from build123d import *

# Parameters (mm, degrees)
BOSS_EXTRUDE1_DEPTH = 60


with BuildPart() as part:
    # Sketch1 → Boss-Extrude1 (new body)
    with BuildSketch(Plane(origin=(0, 0, 0), x_dir=(1, 0, 0), z_dir=(0, 1, 0))):
        with BuildLine():
            Line((-38.729833462, -10), (-20.877867157, -79.140368196))
            Line((-20.877867157, -79.140368196), (-44.722080497, -147.638269612))
            ThreePointArc((-44.722080497, -147.638269612), (-42.5, -153.612159322), (-36.215419503, -152.549592626))
            Line((-36.215419503, -152.549592626), (15.138321986, -93.070241293))
            ThreePointArc((15.138321986, -93.070241293), (17.71723932, -89.278977901), (19.364916731, -85))
            Line((19.364916731, -85), (38.729833462, -10))
            ThreePointArc((38.729833462, -10), (0, 40), (-38.729833462, -10))
        make_face()
    extrude(amount=BOSS_EXTRUDE1_DEPTH)


solid = part.part
Geometry: final body of the model. Coordinates: model frame, mm. A direction names the side the tool comes from. Give positions to 0.01 mm unless a question says otherwise; leave off trailing zeros. Write each loop counter-clockwise with the first axis right and the second up, starting at its lowest first coordinate (ties: lowest second). Pieces come first, ordered by that corner, then holes. Notation, with made-up numbers: M -24,55 L 15,55 A19 ccw 15,82 Z; hole C 9.25,-39.5 d5. An arc over 180 degrees is marked long. Answer in a Markdown table with one row per item. Add a question column.
(1) Section B-B on z = 0. Return loops of the section in (x, y).
(2) Reachability of faces 1 (the flat face through (-29.929, 29.58, 44.086)), 2 (the cylindrical face through (1.021, 29.58, -39.987)) from +Z, -Z, +X, -X, +Y, -Y: full face, straight path, thin tool, end or side. Return the list, or none.
(3) Section C-C on x = 32. Return loops of the section in (y, z), and give its area (3 significant figures).
(4) Section A-A on y = 9.5. Return loops of the section in (x, z).
(5) Mould query, pull axis Z, two halves, no side actions, for faces 3 (the cylindrical face through (17.687, 29.58, 89.336)), 4 (the flat face through (-32.633, 29.58, 112.91)), 5 (the flat face through (-3, 60, 34)). Classes: +Z half, -Z half, draft (parallel to the pull), parting line (faces both ways), or undercut.
(6) Ray query, line 1 (X direction, y = 57, z = 1.5); line 2 (X direction, y = 56, z = -8); line 3 (Z direction, x = 16, y = 43). Return the intervals inside material, ascending.
(7) First-contact query: pin 1 (8 mm diameter, centred on y = 29, z = 133, fed in from +X); pin 2 (1 mm diameter, centred on y = 18.5, z = 66, fed in from -X); pin 3 (12 mm diameter, centred on x = 17.5, y = 41.5, fed in from +Z). Flat tips, straight axial feed; report the tip coordinate or a pass-through.
Result set:
| question | item | result |
|---|---|---|
| 1 | outline | M -40,0 L 40,0 L 40,60 L -40,60 Z |
| 2 | face 1 | -X, +Y, -Y |
| 2 | face 2 | +Y, -Y |
| 3 | outline | M 0,-24 L 60,-24 L 60,36.06 L 0,36.06 Z |
| 3 | area | 3,600 mm^2 |
| 4 | outline | M -44.72,147.64 L -20.88,79.14 L -38.73,10 A40 ccw long 38.73,10 L 19.36,85 A20 ccw 15.14,93.07 L -36.22,152.55 A5 ccw Z |
| 5 | face 3 | +Z half |
| 5 | face 4 | undercut |
| 5 | face 5 | draft |
| 6 | line 1 | x = -39.97 to 39.97 |
| 6 | line 2 | x = -39.19 to 39.19 |
| 6 | line 3 | z = -36.66 to 92 |
| 7 | pin 1 | stops at x = -15.88 |
| 7 | pin 2 | stops at x = -24.4 |
| 7 | pin 3 | stops at z = 97.28 |
